The model under review builds one solid part; all positions refer to its coordinate system, in mm. Face numbers are marked on the shaded views. A direction names the side the tool comes from. Give positions to 0.01 mm unless a question says otherwise; leave off trailing zeros. Loops run counter-clockwise (first coordinate to the right, second up) from the corner with the lowest first, then second, coordinate; pieces in that order, holes last. Notation, with made-up numbers: (-1, -6) - (27, -6) arc R25 ccw to (27, 21) - close; hole circle Ø1 at (49, -18.75). An arc over 180 degrees is marked (long way). Answer as a JSON object with one key per item and string values.
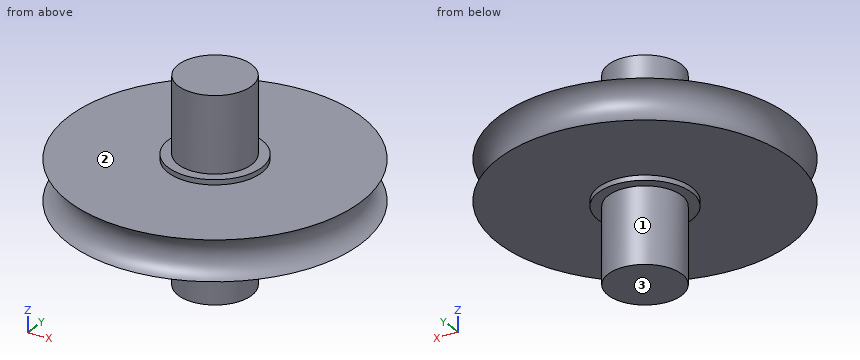
from build123d import *

# Parameters (mm, degrees)
F0_R     = 7.3008019747
F1_DEPTH = 20
F0_R_2   = 9.3008019747
F2_DEPTH = 5
F0_R_3   = 29.0307788443
F3_DEPTH = 4


with BuildPart() as f1:
    # F0 (on Top) → F1 (new body, symmetric)
    with BuildSketch(Plane.XY):
        Circle(F0_R)
    extrude(amount=F1_DEPTH, both=True)

    # F0 (on Top) → F2 (join, symmetric)
    with BuildSketch(Plane.XY):
        Circle(F0_R_2)
        Circle(F0_R, mode=Mode.SUBTRACT)
    extrude(amount=F2_DEPTH, both=True)

    # F0 (on Top) → F3 (join, symmetric)
    with BuildSketch(Plane.XY):
        Circle(F0_R_3)
        Circle(F0_R_2, mode=Mode.SUBTRACT)
    extrude(amount=F3_DEPTH, both=True)

    # F5: sweep along a path in F5_path
    with BuildLine(Plane(origin=(29.0307788443, 0, 4), x_dir=(0, -1, 0), z_dir=(0, 0, -1))) as f5_path:
        CenterArc((0, 29.0307788443), 29.0307788443, 0, 360)
    # F4 (on Right) → F5 (sweep, cut)
    with BuildSketch(Plane.YZ):
        with BuildLine():
            Line((-29.0307788443, 4), (-29.0307788443, -4))
            ThreePointArc((-29.0307788443, -4), (-26.0956077828, 0), (-29.0307788443, 4))
        make_face()
    sweep(path=f5_path.line, mode=Mode.SUBTRACT)


solid = f1.part
Q1. To check wall thickness, follow probe 1 along Z at (x, y) = (-12.5, 1); probe 2 along Z at (x, y) = (26.5, 2); probe 3 along X at (y, z) = (16, 3.5). State the ranges of each line that lie inside material, in increasing order. Write a range as [from, to].
Results:
{"probe 1": "z = [-4, 4]", "probe 2": "z = [-4, -1.95], [1.95, 4]", "probe 3": "x = [-22.95, 22.95]"}
Q2. Consider section A-A, the plane x = 0. State the section outline as (y, z) points, plus the area to 3 significant figures.
Results:
{"outline": "(-29.03, -4) - (-9.3, -4) - (-9.3, -5) - (-7.3, -5) - (-7.3, -20) - (7.3, -20) - (7.3, -5) - (9.3, -5) - (9.3, -4) - (29.03, -4) arc R4.19 cw to (29.03, 4) - (9.3, 4) - (9.3, 5) - (7.3, 5) - (7.3, 20) - (-7.3, 20) - (-7.3, 5) - (-9.3, 5) - (-9.3, 4) - (-29.03, 4) arc R4.19 cw to start", "area": "905 mm^2"}
Q3. Clearance check with flat-ended pins moving along their axes: pin 1 Ø8 at (x, y) = (-9, -7.5) entering from +Z; pin 2 Ø2 at (y, z) = (-1, -4) entering from +X; pin 3 Ø12 at (x, y) = (17, -19.5) entering from -Z. State where each tip first meets the part, or that it passes through.
Results:
{"pin 1": "stops at z = 5", "pin 2": "stops at x = 29.03", "pin 3": "stops at z = -4"}
Q4. Consider section D-D, the plane z = 0.5. State the section outline as (x, y) points, plus the area to 3 significant figures.
Results:
{"outline": "circle Ø52.25 at (0, 0)", "area": "2,140 mm^2"}
Q5. For the marked faces 1, 2 and 3, list the 3-axis set-ups (+Z, -Z, +X, -X, +Y, -Y) from which the entire face can be reached by the end or side of a thin tool; tool diameter is ignored.
Results:
{"face 1": "-Z", "face 2": "+Z", "face 3": "-Z, +X, -X, +Y, -Y"}
Q6. Consider section C-C, the plane z = 7. State the section outline as (x, y) points, plus the area to 3 significant figures.
Results:
{"outline": "circle Ø14.6 at (0, 0)", "area": "167 mm^2"}
